Model file for the job. Use its own axes, mm. Face numbers are marked on the shaded views. A direction names the side the tool comes from. Coordinates: 2 decimals unless noted, no trailing zeros. Order: outer loops, then holes, each group sorted by start corner. A loop starts at its lowest first (then second) coordinate and runs counter-clockwise, first axis right, second up. Notation, with made-up numbers: M 64,44 L 97,44 A13 ccw 97,65 Z; hole C 14,66 d1. An arc over 180 degrees is marked long. Return JSON: item names as keys, results as strings.
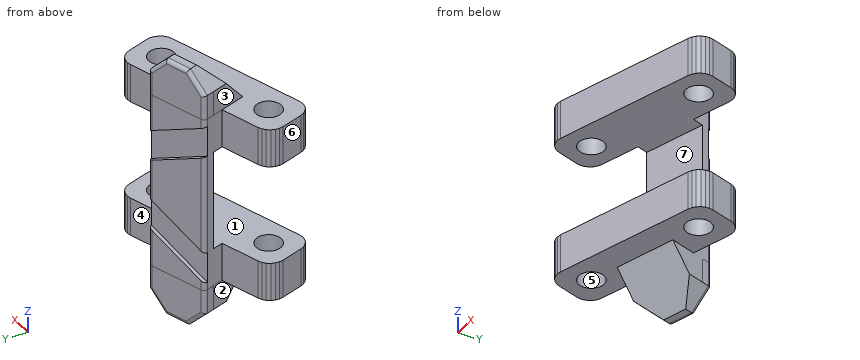
```python
from build123d import *

# Parameters (mm, degrees)
MODEL_R             = 1.665
BOSS_EXTRUDE1_DEPTH = 5
SKETCH2_W           = 8.310460331
SKETCH2_H           = 5
BOSS_EXTRUDE2_DEPTH = 1.5
BOSS_EXTRUDE3_DEPTH = 1.5
BOSS_EXTRUDE4_DEPTH = 5.68
BOSS_EXTRUDE5_DEPTH = 8.31
CUT_EXTRUDE1_DEPTH  = 0.5
CHAMFER1_SIZE       = 2.5
FILLET1_R           = 0.5


with BuildPart() as part:
    # Model → Boss-Extrude1 (new body)
    with BuildSketch(Plane.XY):
        Polygon((17.1125, 65.2434), (16.6413, 65.0186), (16.2442, 64.6796), (15.9485, 64.2493), (15.7742, 63.7571), (15.7333, 63.2366), (15.8284, 62.7233), (16.7555, 59.8701), (16.9802, 59.3988), (17.3193, 59.0018), (17.7496, 58.7061), (18.2418, 58.5318), (18.7623, 58.4909), (19.2756, 58.586), (37.3457, 64.4573), (37.8169, 64.6821), (38.214, 65.0212), (38.5097, 65.4515), (38.684, 65.9436), (38.7249, 66.4641), (38.6298, 66.9775), (37.7027, 69.8306), (37.478, 70.3019), (37.1389, 70.6989), (36.7086, 70.9946), (36.2164, 71.1689), (35.6959, 71.2099), (35.1826, 71.1147), align=None)
        with Locations((34.8376, 67.3225)):
            Circle(MODEL_R, mode=Mode.SUBTRACT)
        with Locations((19.6206, 62.3782)):
            Circle(MODEL_R, mode=Mode.SUBTRACT)
    boss_extrude1 = extrude(amount=BOSS_EXTRUDE1_DEPTH)

    # Sketch2 → Boss-Extrude2 (add)
    with BuildSketch(Plane(origin=(-17.540388664, 53.984054163, 0), x_dir=(0.9510570020345874, 0.3090154994186907, 0), z_dir=(-0.3090154994186907, 0.9510570020345874, 0))):
        with Locations((45.9361937, -2.5)):
            Rectangle(SKETCH2_W, SKETCH2_H)
    boss_extrude2 = extrude(amount=BOSS_EXTRUDE2_DEPTH)

    # Sketch3 → Boss-Extrude3 (add)
    with BuildSketch(Plane(origin=(-18.003911914, 55.410639666, 0), x_dir=(0.9510570020345874, 0.30901549941869066, 0), z_dir=(-0.30901549941869066, 0.9510570020345874, 0))):
        Polygon((41.780963534, 0), (41.780963534, -5), (41.780963534, -11.5), (50.091423865, -11.5), (50.091423865, -5), (50.091423865, 0), align=None)
    boss_extrude3 = extrude(amount=BOSS_EXTRUDE3_DEPTH)

    # Mirror4: Boss-Extrude3 across plane
    add(boss_extrude3.mirror(Plane.XY.offset(11.5)))

    # Mirror5: Boss-Extrude2 across plane
    add(boss_extrude2.mirror(Plane.XY.offset(11.5)))

    # Mirror8: Boss-Extrude1 across plane
    add(boss_extrude1.mirror(Plane.XY.offset(11.5)))

    # Sketch5 → Boss-Extrude4 (add)
    with BuildSketch(Plane(origin=(0, 0, 0), x_dir=(-1, 0, 0), z_dir=(0, 0, -1))):
        Polygon((-29.172364246, 72.316251531), (-29.635887495, 70.889666028), (-21.732166007, 68.321604978), (-21.268642758, 69.748190481), align=None)
    boss_extrude4 = extrude(amount=BOSS_EXTRUDE4_DEPTH)

    # Mirror9: Boss-Extrude4 across plane
    add(boss_extrude4.mirror(Plane.XY.offset(11.5)))

    # Sketch7 → Boss-Extrude5 (add)
    with BuildSketch(Plane(origin=(47.639799409, 15.479026362, 0), x_dir=(0, 0, -1), z_dir=(0.9510570020345875, 0.3090154994186908, 0))):
        Polygon((5.68, 58.262164673), (0, 58.262164673), (0, 53.262164673), align=None)
    boss_extrude5 = extrude(amount=-BOSS_EXTRUDE5_DEPTH)

    # Mirror10: Boss-Extrude5 across plane
    add(boss_extrude5.mirror(Plane.XY.offset(11.5)))

    # Sketch8 → Cut-Extrude1 (cut)
    with BuildSketch(Plane(origin=(-18.467435163, 56.837225169, 0), x_dir=(0.9510570020345874, 0.30901549941869066, 0), z_dir=(-0.30901549941869066, 0.9510570020345874, 0))):
        Polygon((45.936193699, -7), (50.091423865, -9), (50.091423865, -5), (41.780963534, -1), (41.780963534, -5), align=None)
    cut_extrude1 = extrude(amount=-CUT_EXTRUDE1_DEPTH, mode=Mode.SUBTRACT)

    # Mirror11: Cut-Extrude1 across plane
    add(cut_extrude1.mirror(Plane.XY.offset(11.5)), mode=Mode.SUBTRACT)

    # Chamfer1
    # the kernel refuses this chamfer: 2.5 mm, written as the material it takes off along each edge
    with BuildSketch(Plane(origin=(27.185639489, 78.430794313, -5.68), x_dir=(0.02615014597757756, 0.008496652042775076, 0.9996219169112968), z_dir=(0.30901549941868806, -0.9510570020345883, 0)), Plane(origin=(23.718890764, 62.207062196, -5.68), x_dir=(-0.026150145977578018, -0.008496652042775138, 0.9996219169112968), z_dir=(-0.30901549941868506, 0.9510570020345892, 0))) as chamfer1_piece_1:
        Polygon((CHAMFER1_SIZE * 0.999621916911, CHAMFER1_SIZE * 0.0274958766106), (-CHAMFER1_SIZE * 0.0274958766106, CHAMFER1_SIZE * 0.999621916911), (0, 0), align=None)
    extrude(amount=14.35841494, mode=Mode.SUBTRACT)
    with BuildSketch(Plane(origin=(23.718890764, 62.207062196, 28.68), x_dir=(-0.026150145977578018, -0.008496652042775138, -0.9996219169112968), z_dir=(-0.30901549941868506, 0.9510570020345892, 0)), Plane(origin=(27.185639489, 78.430794313, 28.68), x_dir=(0.02615014597757756, 0.008496652042775076, -0.9996219169112968), z_dir=(0.30901549941868806, -0.9510570020345883, 0))) as chamfer1_piece_2:
        Polygon((CHAMFER1_SIZE * 0.999621916911, -CHAMFER1_SIZE * 0.0274958766106), (-CHAMFER1_SIZE * 0.0274958766106, -CHAMFER1_SIZE * 0.999621916911), (0, 0), align=None)
    extrude(amount=14.35841494, mode=Mode.SUBTRACT)

    # Fillet1
    fillet1_edges = [part.edges().sort_by_distance(p)[0] for p in [
        (29.172364246, 72.316251531, 0.91),
        (21.268642758, 69.748190481, 11.5),
        (29.172364246, 72.316251531, 11.5),
        (21.268642758, 69.748190481, 24.09),
        (21.268642758, 69.748190481, -1.09),
        (25.220503502, 71.032221006, 28.68),
        (29.172364246, 72.316251531, 22.09),
        (27.983542993, 71.929982157, 27.43),
        (22.45746401, 70.134459856, 27.43),
        (25.220503502, 71.032221006, -5.68),
        (22.45746401, 70.134459856, -4.43),
        (27.983542993, 71.929982157, -4.43),
    ]]
    fillet(fillet1_edges, radius=FILLET1_R)


solid = part.part
```
Item 1: Pull direction X, two halves, no side cores. Call the marked faces 5, 6 and 7: +X half, -X half, draft (parallel to the pull), parting line (faces both ways), or undercut.
Check result:
{"face 5": "undercut", "face 6": "-X half", "face 7": "+X half"}
Item 2: Saw through at D-D (z = 2). Count the separate pieces of the cut face and the enclosed holes in it, and give its area (3 significant figures).
Check result:
{"separate pieces": "1", "enclosed holes": "2", "area": "164 mm2"}
Item 3: 3-axis set-ups, long thin cutter, end or side, ignore diameter. For the marked faces 1, 2, 3 and 4: which of +Z, -Z, +X, -X, +Y, -Y reach the whole face in a straight line?
Check result:
{"face 1": "+X, -Y", "face 2": "-Z, -X, -Y", "face 3": "+Z, -X, -Y", "face 4": "+Z, -Z, +Y"}
Item 4: Drop flat-ended pins along their axis: pin 1 Ø6.5 at (x, y) = (25.5, 67.5) entering from +Z; pin 2 Ø2.5 at (x, y) = (19.62, 62.38) entering from -Z; pin 3 Ø5.5 at (x, y) = (34.84, 67.32) entering from -Z; pin 4 Ø4 at (x, y) = (35.5, 68) entering from +Z. Give the stop position or say it passes through.
Check result:
{"pin 1": "stops at z = 28.68", "pin 2": "passes through", "pin 3": "stops at z = 0", "pin 4": "stops at z = 23"}
Item 5: Wall check: line 1 (Y direction, x = 34, z = 21); line 2 (X direction, y = 68, z = 3); line 3 (Y direction, x = 35.25, z = 22.5). Give the ranges that are in metal, low to high.
Check result:
{"line 1": "y = 63.37 to 65.88, 68.76 to 70.73", "line 2": "x = 21.84 to 33.32, 36.36 to 38.3", "line 3": "y = 63.78 to 65.71, 68.94 to 71.13"}
Item 6: Saw through at B-B (x = 20.75). Write the cut outline in (y, z), and give its area (3 significant figures).
Check result:
{"outline": "M 59.07,0 L 61.15,0 L 61.15,5 L 59.07,5 Z; M 59.07,18 L 61.15,18 L 61.15,23 L 59.07,23 Z; M 63.6,0 L 66.43,0 L 66.43,5 L 63.6,5 Z; M 63.6,18 L 66.43,18 L 66.43,23 L 63.6,23 Z", "area": "49.1 mm2"}
Item 7: Saw through at A-A (x = 32.75). Write the cut outline in (y, z), and give its area (3 significant figures).
Check result:
{"outline": "M 62.96,0 L 70.32,0 L 70.32,5 L 62.96,5 Z; M 62.96,18 L 70.32,18 L 70.32,23 L 62.96,23 Z", "area": "73.6 mm2"}
